Geometry: final body of the model. Coordinates: model frame, mm. Face numbers are marked on the shaded views. Coordinates: 2 decimals unless noted, no trailing zeros. Loops run counter-clockwise (first coordinate to the right, second up) from the corner with the lowest first, then second, coordinate; pieces in that order, holes last. Notation, with made-up numbers: M 77,23 L 102,23 A9 cw 102,29 Z; hole C -39.75,-39.75 d7. An arc over 180 degrees is marked long. Write item = value, one per line. Start each with the question number.
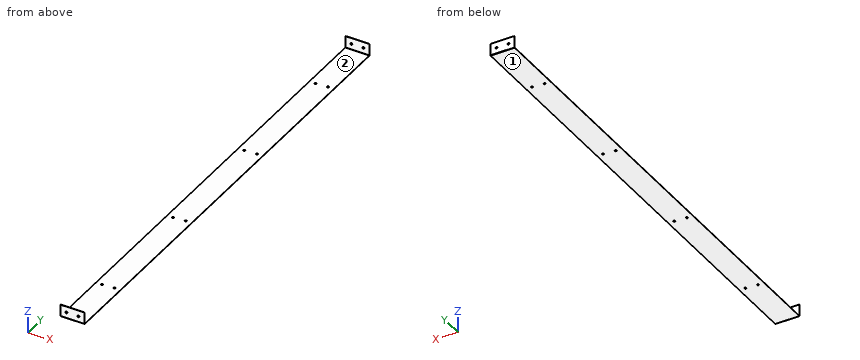
Autodesk Inventor part; units mm, degrees
ref_plane "YZ Plane" through (0, 0, 0) normal (1, 0, 0) x (0, 1, 0)
ref_plane "XZ Plane" through (0, 0, 0) normal (0, 1, 0) x (-1, 0, 0)
ref_plane "XY Plane" through (0, 0, 0) normal (0, 0, 1) x (1, 0, 0)
sketch "Sketch1" plane through (0, 0, 0) normal (0, 0, 1) x (1, 0, 0)
  line L0 (0, 0) -> (50, 0)
  line L1 (50, 0) -> (50, 1002)
  line L2 (50, 1002) -> (0, 1002)
  line L3 (0, 1002) -> (0, 0)
  dimension "d0" = 50
  dimension "d1" = 1002
extrude "Plate1" add sketch "Sketch1" along normal blind 0.5
sketch "Sketch2" plane through (0, 0, 0.5) normal (0, 0, 1) x (1, 0, 0)
  circle A0 centre (12.5, 125) radius 2
  line L0 (50, 0) -> (0, 0)
  line L1 (0, 0) -> (0, 1002)
  circle A1 centre (12.5, 375) radius 2
  circle A2 centre (12.5, 625) radius 2
  circle A3 centre (12.5, 875) radius 2
  circle A4 centre (37.5, 877) radius 2
  line L2 (50, 1002) -> (50, 0)
  line L3 (0, 1002) -> (50, 1002)
  circle A5 centre (37.5, 627) radius 2
  circle A6 centre (37.5, 377) radius 2
  circle A7 centre (37.5, 127) radius 2
  dimension "d3" = 4
  dimension "d4" = 125
  dimension "d5" = 12.5
  dimension "d6" = 4
  dimension "d7" = 250
  dimension "d8" = 12.5
  dimension "d9" = 4
  dimension "d10" = 250
  dimension "d11" = 12.5
  dimension "d12" = 4
  dimension "d13" = 250
  dimension "d14" = 12.5
  dimension "d15" = 4
  dimension "d16" = 12.5
  dimension "d17" = 125
  dimension "d18" = 4
  dimension "d19" = 250
  dimension "d20" = 12.5
  dimension "d21" = 4
  dimension "d22" = 250
  dimension "d23" = 12.5
  dimension "d24" = 4
  dimension "d25" = 250
  dimension "d26" = 12.5
hole "Hole1" at (12.5, 875, 0.5) at (37.5, 877, 0.5) at (37.5, 627, 0.5) at (12.5, 625, 0.5) at (37.5, 377, 0.5) at (12.5, 375, 0.5) at (37.5, 127, 0.5) at (12.5, 125, 0.5) direction (0, 0, -1) diameter 4 end through all
sketch "Sketch3" plane through (0, 1001.5, 0) normal (0, 1, 0) x (-1, 0, 0)
  line L0 (-50, 0) -> (0, 0)
  line L1 (0, 0) -> (0, 25)
  line L2 (0, 25) -> (-50, 25)
  line L3 (-50, 25) -> (-50, 0)
edge flange "Flange1" height 25 angle 90 thickness 0.5 bend radius 0.5 thickness toward (0, 1, 0) relief tear relief width 0.5 relief depth 0.25 edges at (25, 1002, 0.5) wall of the first edge with corners at (50, 1001.5, 0) (0, 1001.5, 0) (0, 1001.5, 25) (50, 1001.5, 25)
bend "Bend1"
corner "Corner1"
sketch "Sketch4" plane through (50, 0.5, 0) normal (0, -1, 0) x (1, 0, 0)
  line L0 (-50, 0) -> (0, 0)
  line L1 (0, 0) -> (0, 25)
  line L2 (0, 25) -> (-50, 25)
  line L3 (-50, 25) -> (-50, 0)
edge flange "Flange2" height 25 angle 90 thickness 0.5 bend radius 0.5 thickness toward (0, -1, 0) relief tear relief width 0.5 relief depth 0.25 edges at (25, 0, 0.5) wall of the first edge with corners at (0, 0.5, 0) (50, 0.5, 0) (50, 0.5, 25) (0, 0.5, 25)
bend "Bend2"
corner "Corner2"
sketch "Sketch5" plane through (0, 1002, 25) normal (0, 1, 0) x (1, 0, 0)
  circle A0 centre (12.5, 12.5) radius 2
  circle A1 centre (37.5, 12.5) radius 2
  line L0 (0, 0) -> (0, 24)
  line L1 (50, 24) -> (50, 0)
  line L2 (50, 0) -> (0, 0)
  point P0 (0, 25)
  dimension "d54" = 4
  dimension "d55" = 4
  dimension "d56" = 12.5
  dimension "d57" = 12.5
  dimension "d58" = 12.5
  dimension "d59" = 12.5
hole "Hole2" at (12.5, 1002, 12.5) at (37.5, 1002, 12.5) direction (0, -1, 0) diameter 4 end through all
equation "\"d0\" = A_width"
equation "\"d3\" = rivet_diameter"
equation "\"d4\" = 0.5 * rivet_displacement"
equation "\"d5\" = 0.25 * A_width"
equation "\"d6\" = rivet_diameter"
equation "\"d7\" = rivet_displacement"
equation "\"d8\" = 0.25 * A_width"
equation "\"d9\" = rivet_diameter"
equation "\"d10\" = rivet_displacement"
equation "\"d11\" = 0.25 * A_width"
equation "\"d12\" = rivet_diameter"
equation "\"d13\" = rivet_displacement"
equation "\"d14\" = 0.25 * A_width"
equation "\"d15\" = rivet_diameter"
equation "\"d16\" = 0.25 * A_width"
equation "\"d17\" = 0.5 * rivet_displacement"
equation "\"d18\" = rivet_diameter"
equation "\"d19\" = rivet_displacement"
equation "\"d20\" = 0.25 * A_width"
equation "\"d21\" = rivet_diameter"
equation "\"d22\" = rivet_displacement"
equation "\"d23\" = 0.25 * A_width"
equation "\"d24\" = rivet_diameter"
equation "\"d25\" = rivet_displacement"
equation "\"d26\" = 0.25 * A_width"
equation "\"d27\" = rivet_diameter"
equation "\"d32\" = Thickness"
equation "\"d54\" = rivet_diameter"
equation "\"d55\" = rivet_diameter"
equation "\"d56\" = 0.25 * A_width"
equation "\"d57\" = 0.25 * A_width"
equation "\"d58\" = 0.25 * A_width"
equation "\"d59\" = 0.25 * A_width"
equation "\"d60\" = rivet_diameter"
equation "\"d65\" = Thickness"
equation "\"d2\" = Thickness"
equation "\"d34\" = BendReliefWidth"
equation "\"d35\" = BendReliefDepth"
equation "\"d36\" = MinimumRemnant"
equation "\"d37\" = TransitionRadius"
equation "\"d38\" = 0.5 * A_width"
equation "\"d40\" = BendRadius"
equation "\"d41\" = CornerReliefSize"
equation "\"d42\" = GapSize"
equation "\"d43\" = JacobiRadiusSize"
equation "\"d44\" = BendReliefWidth"
equation "\"d45\" = BendReliefDepth"
equation "\"d46\" = MinimumRemnant"
equation "\"d47\" = TransitionRadius"
equation "\"d48\" = 0.5 * A_width"
equation "\"d50\" = BendRadius"
equation "\"d51\" = CornerReliefSize"
equation "\"d52\" = GapSize"
equation "\"d53\" = JacobiRadiusSize"
equation "\"BendRadius\" = Thickness"
equation "\"BendReliefWidth\" = Thickness"
equation "\"BendReliefDepth\" = 0.5 * Thickness"
equation "\"CornerReliefSize\" = 4 * Thickness"
equation "\"MinimumRemnant\" = 2 * Thickness"
equation "\"TransitionRadius\" = BendRadius"
equation "\"JacobiRadiusSize\" = BendRadius"
equation "\"GapSize\" = Thickness"
equation "\"A_width\" = 50"
equation "\"l___________\" = 0"
equation "\"l__________\" = 0"
equation "\"l_________\" = 0"
equation "\"rivet_diameter\" = 4"
equation "\"rivet_displacement\" = 250"
equation "\"l________\" = 0"
equation "\"plate_thickness\" = 2"
properties part number "A1_BeamCoverPlate"
Item 1: Pull-direction query (Y, two-part tool) for the marked faces 1 and 2; classes: released by +Y, released by -Y, zero draft, split by the parting line, or undercut.
Item 2: Section query A-A (z = 5). Return the cut outline in (x, y).
Item 3: First-contact query: pin 1 (5 mm diameter, centred on x = 43, y = 419.5, fed in from +Z); pin 2 (2.5 mm diameter, centred on x = 12.5, z = 12.5, fed in from -Y). Flat tips, straight axial feed; report the tip coordinate or a pass-through.
Item 4: Line query: line 1 (X direction, y = 1001.7, z = 12.5); line 2 (Y direction, x = 37.5, z = 0.4); line 3 (Y direction, x = 12.5, z = 0.2). Output: solid intervals per line, ascending. Write a range as from..to.
Item 5: Section query B-B (y = 598). Return the cut outline in (x, z).
Verdict:
q1.face_1 = zero draft
q1.face_2 = undercut
q2.outline = M 0,0 L 50,0 L 50,0.5 L 0,0.5 Z; M 0,1001.5 L 50,1001.5 L 50,1002 L 0,1002 Z
q3.pin_1 = 0.5
q3.pin_2 = through
q4.line_1 = 0..10.5, 14.5..35.5, 39.5..50
q4.line_2 = 0.2..125, 129..375, 379..625, 629..875, 879..1001.8
q4.line_3 = 0.4..123, 127..373, 377..623, 627..873, 877..1001.6
q5.outline = M 0,0 L 50,0 L 50,0.5 L 0,0.5 Z
